from build123d import *

# Parameters (mm, degrees)
SKETCH1_R                                       = 35
BOSS_EXTRUDE1_DEPTH                             = 6.35
SKETCH2_W                                       = 25.4
SKETCH2_H                                       = 69.5
SKETCH2_W_2                                     = 14.7
SKETCH2_H_2                                     = 52.8
BOSS_EXTRUDE2_DEPTH                             = 15.578435
CSK_FOR_M8_FLAT_HEAD_MACHINE_SCREW1_D           = 9
CSK_FOR_M8_FLAT_HEAD_MACHINE_SCREW1_DEPTH       = 17.5
CSK_FOR_M8_FLAT_HEAD_MACHINE_SCREW1_CSINK_D     = 17.3
CSK_FOR_M8_FLAT_HEAD_MACHINE_SCREW1_CSINK_ANGLE = 90
CSK_FOR_M8_FLAT_HEAD_MACHINE_SCREW1_TIP         = 2.703872786
SKETCH6_W                                       = 15.578435
SKETCH6_H                                       = 11.9
BOSS_EXTRUDE3_DEPTH                             = 25.572145
SKETCH7_W                                       = 15.578435
SKETCH7_H                                       = 11.9
BOSS_EXTRUDE4_DEPTH                             = 10.937286
SKETCH8_R                                       = 2.5273
CUT_EXTRUDE1_DEPTH                              = 7
SKETCH9_W                                       = 10
SKETCH9_H                                       = 11.9
BOSS_EXTRUDE5_DEPTH                             = 4.972688
SKETCH10_R                                      = 2.5273
CUT_EXTRUDE2_DEPTH                              = 7
SKETCH11_W                                      = 5.3384196
SKETCH11_H                                      = 10
BOSS_EXTRUDE6_DEPTH                             = 5.35
SKETCH12_W                                      = 10
SKETCH12_H                                      = 10
SKETCH12_W_2                                    = 7.789222
SKETCH12_H_2                                    = 5
BOSS_EXTRUDE7_DEPTH                             = 11.85
SKETCH13_R                                      = 2.5273
CUT_EXTRUDE3_DEPTH                              = 7
SKETCH14_W                                      = 5.35
SKETCH14_H                                      = 10
CUT_EXTRUDE4_DEPTH                              = 5.33842


with BuildPart() as part:
    # Sketch1 → Boss-Extrude1 (new body)
    with BuildSketch(Plane.XY):
        Circle(SKETCH1_R)
    extrude(amount=BOSS_EXTRUDE1_DEPTH)

    # Sketch2 → Boss-Extrude2 (add)
    with BuildSketch(Plane(origin=(0, 0, 0), x_dir=(-1, 0, 0), z_dir=(0, 0, -1))):
        Rectangle(SKETCH2_W, SKETCH2_H)
        with Locations((0, -3)):
            Rectangle(SKETCH2_W_2, SKETCH2_H_2, mode=Mode.SUBTRACT)
    extrude(amount=BOSS_EXTRUDE2_DEPTH)

    # CSK for M8 Flat Head Machine Screw1
    with Locations(Plane.XY.offset(6.35)):
        with Locations((0, -3)):
            CounterSinkHole(CSK_FOR_M8_FLAT_HEAD_MACHINE_SCREW1_D / 2, CSK_FOR_M8_FLAT_HEAD_MACHINE_SCREW1_CSINK_D / 2, depth=CSK_FOR_M8_FLAT_HEAD_MACHINE_SCREW1_DEPTH, counter_sink_angle=CSK_FOR_M8_FLAT_HEAD_MACHINE_SCREW1_CSINK_ANGLE)
            with Locations((0, 0, -(CSK_FOR_M8_FLAT_HEAD_MACHINE_SCREW1_DEPTH + CSK_FOR_M8_FLAT_HEAD_MACHINE_SCREW1_TIP / 2))):  # 118° drill point
                Cone(0, CSK_FOR_M8_FLAT_HEAD_MACHINE_SCREW1_D / 2, CSK_FOR_M8_FLAT_HEAD_MACHINE_SCREW1_TIP, mode=Mode.SUBTRACT)

    # Sketch6 → Boss-Extrude3 (add)
    with BuildSketch(Plane(origin=(12.7, 0, 0), x_dir=(0, 0, -1), z_dir=(1, 0, 0))):
        with Locations((7.7892175, 28.8)):
            Rectangle(SKETCH6_W, SKETCH6_H)
    extrude(amount=BOSS_EXTRUDE3_DEPTH)

    # Sketch7 → Boss-Extrude4 (add)
    with BuildSketch(Plane.ZY.offset(12.7)):
        with Locations((-7.7892175, 28.8)):
            Rectangle(SKETCH7_W, SKETCH7_H)
    extrude(amount=BOSS_EXTRUDE4_DEPTH)

    # Sketch8 → Cut-Extrude1 (cut)
    with BuildSketch(Plane(origin=(0, 34.75, 0), x_dir=(1, 0, 0), z_dir=(0, 1, 0))):
        with Locations((-18.637286, 9.228435)):
            Circle(SKETCH8_R)
    extrude(amount=-CUT_EXTRUDE1_DEPTH, mode=Mode.SUBTRACT)

    # Sketch9 → Boss-Extrude5 (add)
    with BuildSketch(Plane(origin=(0, 0, -15.578435), x_dir=(-1, 0, 0), z_dir=(0, 0, -1))):
        with Locations((-33.272145, 28.8)):
            Rectangle(SKETCH9_W, SKETCH9_H)
    extrude(amount=BOSS_EXTRUDE5_DEPTH)

    # Sketch10 → Cut-Extrude2 (cut)
    with BuildSketch(Plane(origin=(0, 34.75, 0), x_dir=(1, 0, 0), z_dir=(0, 1, 0))):
        with Locations((33.272145, 14.201123)):
            Circle(SKETCH10_R)
    extrude(amount=-CUT_EXTRUDE2_DEPTH, mode=Mode.SUBTRACT)

    # Sketch11 → Boss-Extrude6 (add)
    with BuildSketch(Plane(origin=(12.7, 0, 0), x_dir=(0, 0, -1), z_dir=(1, 0, 0))):
        with Locations((18.2476448, -8.175)):
            Rectangle(SKETCH11_W, SKETCH11_H)
    extrude(amount=-BOSS_EXTRUDE6_DEPTH)

    # Sketch12 → Boss-Extrude7 (add)
    with BuildSketch(Plane(origin=(12.7, 0, 0), x_dir=(0, 0, -1), z_dir=(1, 0, 0))):
        with Locations((15.9168546, -8.175)):
            Rectangle(SKETCH12_W, SKETCH12_H)
        with Locations((11.683824, 10.825)):
            Rectangle(SKETCH12_W_2, SKETCH12_H_2)
        with Locations((11.683824, -27.175)):
            Rectangle(SKETCH12_W_2, SKETCH12_H_2)
    extrude(amount=BOSS_EXTRUDE7_DEPTH)

    # Sketch13 → Cut-Extrude3 (cut)
    with BuildSketch(Plane(origin=(24.55, 0, 0), x_dir=(0, 0, -1), z_dir=(1, 0, 0))):
        with Locations((15.4092126, -8.175)):
            Circle(SKETCH13_R)
    extrude(amount=-CUT_EXTRUDE3_DEPTH, mode=Mode.SUBTRACT)

    # Sketch14 → Cut-Extrude4 (cut)
    with BuildSketch(Plane(origin=(0, 0, -20.9168546), x_dir=(-1, 0, 0), z_dir=(0, 0, -1))):
        with Locations((-10.025, -8.175)):
            Rectangle(SKETCH14_W, SKETCH14_H)
    extrude(amount=-CUT_EXTRUDE4_DEPTH, mode=Mode.SUBTRACT)


solid = part.part
Design review of the part built by this model. Coordinates are the model's own, in mm. A direction names the side the tool comes from. Give positions to 0.01 mm unless a question says otherwise; leave off trailing zeros. Loops run counter-clockwise (first coordinate to the right, second up) from the corner with the lowest first, then second, coordinate; pieces in that order, holes last. Notation, with made-up numbers: M 74.25,-17.5 L 105.25,-17.5 A16 cw 105.25,2.5 Z; hole C 53,84 d11. An arc over 180 degrees is marked long. One line per question, with ' | ' between items. Start each with the question number.
1. Insertion check: P1, Ø8, axis at x = 33.27, z = -14.2, coming from the -Y side; P2, Ø4, axis at x = 23, z = -15, coming from the -Y side (3 decimals); P3, Ø4.5, axis at x = -1.5, z = -4.5, coming from the -Y side; P4, Ø10, axis at y = 0, z = -2, coming from the -X side. Each pin has a flat end and moves straight along its axis. Give the tip position at first contact, or say it passes through.
2. Add section A-A (x = 20). Write out the cut boundary in (y, z) (3 decimals), plus the area to 3 significant figures.
3. The part is to be moulded in two halves that separate along Y. For faces 1 (the face through (19, 13.325, -12)), 2 (the face through (19, -29.675, -12)), 3 (the face through (33, 27.75, -14)), 4 (the face through (24.55, -8.1, -18.1)), say which applies: released by +Y, released by -Y, zero draft, split by the parting line, or undercut.
4. Add section B-B (x = 0). Write out the cut boundary in (y, z), plus the area to 3 significant figures.
5. To check wall thickness, follow L1, parallel to X at y = -13.5, z = -13.75; L2, parallel to X at y = 9.5, z = -10.25; L3, parallel to Y at x = -7, z = -2.5. State the ranges of each line that lie inside material, in increasing order.
6. For faces 5 (the face through (-12.7, -6, -8)), 6 (the face through (-16.227, 31.299, -9.988)), 7 (the face through (19, 8.325, -12)), list the 3-axis set-ups (+Z, -Z, +X, -X, +Y, -Y) from which the entire face can be reached by the end or side of a thin tool; tool diameter is ignored.
7. Add section C-C (y = 30.5). Write out the cut boundary in (x, z), plus the area to 3 significant figures.
8. Add section D-D (y = 22). Write out the cut boundary in (x, z), plus the area to 3 significant figures.
Worked out:
1) P1: stops at y = 22.85 | P2: stops at y = -29.675 | P3: stops at y = -34.75 | P4: stops at x = -35
2) outline: M -29.675,-15.578 L -24.675,-15.578 L -24.675,-7.789 L -29.675,-7.789 Z; M -28.723,0 L 22.85,0 L 22.85,-15.578 L 34.75,-15.578 L 34.75,0 L 28.723,0 L 28.723,6.35 L -28.723,6.35 Z; M -13.175,-20.917 L -3.175,-20.917 L -3.175,-10.917 L -13.175,-10.917 Z; M 8.325,-15.578 L 13.325,-15.578 L 13.325,-7.789 L 8.325,-7.789 Z; hole C -8.175,-15.409 d5.055 | area: 708 mm²
3) face 1: undercut | face 2: released by -Y | face 3: released by +Y | face 4: zero draft
4) outline: M -35,0 L -34.75,0 L -34.75,-15.58 L -29.4,-15.58 L -29.4,0 L -7.5,0 L -7.5,2.2 L -11.65,6.35 L -35,6.35 Z; M 1.5,0 L 23.4,0 L 23.4,-15.58 L 34.75,-15.58 L 34.75,0 L 35,0 L 35,6.35 L 5.65,6.35 L 1.5,2.2 Z | area: 630 mm²
5) L1: x = -12.7 to -7.35, 7.35 to 12.7 | L2: x = -12.7 to -7.35, 7.35 to 24.55 | L3: y = -34.75 to -29.4, 23.4 to 34.75
6) face 5: -Z, -X, -Y | face 6: +Y | face 7: -Z, +X
7) outline: M -23.64,-15.58 L 28.27,-15.58 L 28.27,-20.55 L 38.27,-20.55 L 38.27,0 L 17.17,0 L 17.17,6.35 L -17.17,6.35 L -17.17,0 L -23.64,0 Z; hole C -18.64,-9.23 d5.05; hole C 33.27,-14.2 d5.05 | area: 1,190 mm²
8) outline: M -27.22,0 L -12.7,0 L -12.7,-15.58 L -7.35,-15.58 L -7.35,0 L 7.35,0 L 7.35,-15.58 L 12.7,-15.58 L 12.7,0 L 27.22,0 L 27.22,6.35 L -27.22,6.35 Z | area: 512 mm²
